Can you work these out from the model? Positions are in its coordinate system, mm. Face numbers are marked on the shaded views. A direction names the side the tool comes from. Coordinates: 2 decimals unless noted, no trailing zeros. Loops run counter-clockwise (first coordinate to the right, second up) from the corner with the lowest first, then second, coordinate; pieces in that order, holes last. Notation, with made-up numbers: M -22,81.25 L 27,81.25 A27 cw 27,108.25 Z; hole C 5,21 d11. An arc over 180 degrees is marked long. Return JSON: item names as keys, results as strings. Group by question number.
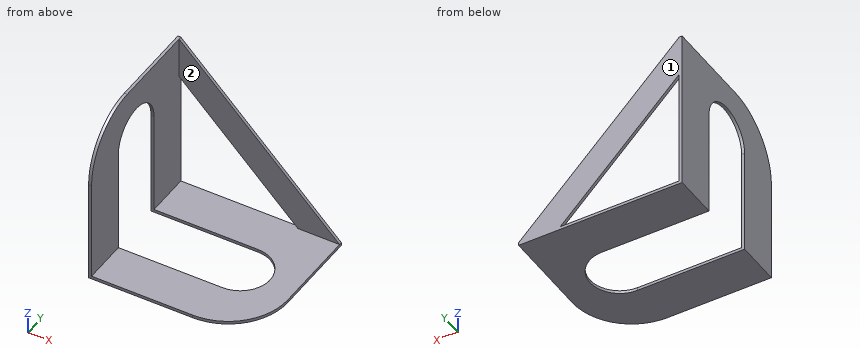
```python
from build123d import *

# Parameters (mm, degrees)
F0_W      = 139.7
F0_H      = 127
F1_DEPTH  = 139.7
F2_W      = 137.16
F2_H      = 137.16
F3_DEPTH  = 124.46
F5_DEPTH  = 25.4
F7_DEPTH  = 25.4
F9_DEPTH  = 25.4
F11_DEPTH = 25.4
F12_R     = 50.8


with BuildPart() as f1:
    # F0 (on Top) → F1 (new body)
    with BuildSketch(Plane.XY):
        with Locations((-69.85, -63.5)):
            Rectangle(F0_W, F0_H)
    extrude(amount=F1_DEPTH)

    # F2 (on face) → F3 (cut)
    with BuildSketch(Plane.XZ.offset(127)):
        with Locations((-68.58, 71.12)):
            Rectangle(F2_W, F2_H)
    extrude(amount=-F3_DEPTH, mode=Mode.SUBTRACT)

    # F4 (on face) → F5 (cut)
    with BuildSketch(Plane.XZ.offset(2.54)):
        Polygon((-6.918556, 178.288981), (-137.16, 139.7), (0, 2.54), (55.803198, 142.750546), align=None)
    extrude(amount=-F5_DEPTH, mode=Mode.SUBTRACT)

    # F6 (on face) → F7 (cut)
    with BuildSketch(Plane.XZ.offset(2.54)):
        Polygon((-137.16, 104.14), (-137.16, 2.54), (-35.56, 2.54), align=None)
    extrude(amount=-F7_DEPTH, mode=Mode.SUBTRACT)

    # F8 (on face) → F9 (cut)
    with BuildSketch(Plane.XY.offset(2.54)):
        with BuildLine():
            Line((-137.16, -38.1), (-137.16, -88.9))
            Line((-137.16, -88.9), (-48.26, -88.9))
            ThreePointArc((-48.26, -88.9), (-22.86, -63.5), (-48.26, -38.1))
            Line((-48.26, -38.1), (-137.16, -38.1))
        make_face()
    extrude(amount=-F9_DEPTH, mode=Mode.SUBTRACT)

    # F10 (on face) → F11 (cut)
    with BuildSketch(Plane.YZ.offset(-137.16)):
        with BuildLine():
            Line((-38.1, 0), (-38.1, 2.54))
            Line((-38.1, 2.54), (-38.1, 91.44))
            ThreePointArc((-38.1, 91.44), (-63.5, 116.84), (-88.9, 91.44))
            Line((-88.9, 91.44), (-88.9, 2.54))
            Line((-88.9, 2.54), (-88.9, 0))
            Line((-88.9, 0), (-38.1, 0))
        make_face()
    extrude(amount=-F11_DEPTH, mode=Mode.SUBTRACT)

    # F12
    f12_edges = [f1.edges().sort_by_distance(p)[0] for p in [
        (0, -127, 1.27),
        (-138.43, -127, 139.7),
    ]]
    fillet(f12_edges, radius=F12_R)


solid = f1.part
```
1) If I drill on line 1 (Z direction, x = -125, y = -119.5); line 2 (X direction, y = -6, z = 131); line 3 (Y direction, x = -49.5, z = 26), over which ranges is the centre line in solid material (lowest first)? Write a range as from..to.
2) For pin 1 (5 mm diameter, centred on x = -61.5, y = -104, fed in from -Z); pin 2 (5 mm diameter, centred on y = -22.5, z = 52, fed in from +X), each with a flat end and sliding along its axis, tell me the tip position at first contact or that it passes through.
3) Suppose I cut it at D-D, the plane y = -86. List the corners of the cut face in (x, z) for me.
4) Suppose I cut it at B-B, the plane z = 39. List the corners of the cut face in (x, y) for me.
5) Suppose I cut it at C-C, the plane z = 109. List the corners of the cut face in (x, y) for me, then the cut area to 3 significant figures.
6) Suppose I cut it at A-A, the plane x = -103.5. List the corners of the cut face in (y, z) for me, then the cut area to 3 significant figures.
7) For the marked faces 1 and 2, which set-ups out of +Z, -Z, +X, -X, +Y, -Y let a thin tool reach every point of the face, with its end or its side?
Returned:
{
 "1": {"line 1": "z = 0..2.54", "line 2": "x = -139.7..-137.16", "line 3": "y = -2.54..0"},
 "2": {"pin 1": "stops at z = 0", "pin 2": "stops at x = -137.16"},
 "3": {"outline": "M -139.7,103.23 L -137.16,103.23 L -137.16,138.75 L -139.7,138.75 Z; M -36.47,0 L -0.95,0 L -0.95,2.54 L -36.47,2.54 Z"},
 "4": {"outline": "M -139.7,-127 L -137.16,-127 L -137.16,-88.9 L -139.7,-88.9 Z; M -139.7,-38.1 L -137.16,-38.1 L -137.16,0 L -139.7,0 Z; M -72.02,-2.54 L -36.46,-2.54 L -36.46,0 L -72.02,0 Z"},
 "5": {"outline": "M -139.7,-122.85 L -137.16,-122.85 L -137.16,-81.85 L -139.7,-81.85 Z; M -139.7,-45.15 L -137.16,-45.15 L -137.16,-2.54 L -106.46,-2.54 L -106.46,0 L -139.7,0 Z", "area": "297 mm²"},
 "6": {"outline": "M -127,0 L -88.9,0 L -88.9,2.54 L -127,2.54 Z; M -38.1,0 L 0,0 L 0,2.54 L -38.1,2.54 Z; M -2.54,70.48 L 0,70.48 L 0,106.04 L -2.54,106.04 Z", "area": "284 mm²"},
 "7": {"face 1": "+Z, -Z, +X, -X, +Y", "face 2": "+Z, +X, -Y"}
}
